```python
from build123d import *

# Parameters (mm, degrees)
SKETCH1_W           = 50.8
SKETCH1_H           = 25.4
BOSS_EXTRUDE1_DEPTH = 2.38125
CUT_EXTRUDE1_REACH  = 6.763
SKETCH2_R           = 3.175


with BuildPart() as part:
    # Sketch1 → Boss-Extrude1 (new body, symmetric)
    with BuildSketch(Plane(origin=(0, 0, 0), x_dir=(1, 0, 0), z_dir=(0, 1, 0))):
        Rectangle(SKETCH1_W, SKETCH1_H)
    extrude(amount=BOSS_EXTRUDE1_DEPTH, both=True)

    # Sketch2 → Cut-Extrude1 (cut, up to next)
    with BuildSketch(Plane(origin=(0, 2.38125, 0), x_dir=(1, 0, 0), z_dir=(0, 1, 0)), mode=Mode.PRIVATE) as cut_extrude1_sk1:
        with Locations((-12.7, 0)):
            Circle(SKETCH2_R)
    cut_extrude1_tool1 = extrude(cut_extrude1_sk1.sketch, amount=-CUT_EXTRUDE1_REACH, mode=Mode.PRIVATE) & part.part
    add(cut_extrude1_tool1.solids().sort_by_distance((-12.7, 2.38125, 0))[0], mode=Mode.SUBTRACT)
    # Sketch2 → Cut-Extrude1 (cut, up to next)
    with BuildSketch(Plane(origin=(0, 2.38125, 0), x_dir=(1, 0, 0), z_dir=(0, 1, 0)), mode=Mode.PRIVATE) as cut_extrude1_sk2:
        with Locations((12.7, 0)):
            Circle(SKETCH2_R)
    cut_extrude1_tool2 = extrude(cut_extrude1_sk2.sketch, amount=-CUT_EXTRUDE1_REACH, mode=Mode.PRIVATE) & part.part
    add(cut_extrude1_tool2.solids().sort_by_distance((12.7, 2.38125, 0))[0], mode=Mode.SUBTRACT)


solid = part.part
```
CAD build for the part. Positions are in the model's coordinates, mm. Coordinates: 2 decimals unless noted, no trailing zeros. Loops run counter-clockwise (first coordinate to the right, second up) from the corner with the lowest first, then second, coordinate; pieces in that order, holes last. Notation, with made-up numbers: (51.5, 50.5) - (95.5, 50.5) arc R24 cw to (95.5, 70.5) - close; hole circle Ø5 at (41.5, 64). An arc over 180 degrees is marked (long way). Return JSON: item names as keys, results as strings.
1. Mould opens along Z. For faces 1 (the flat face through (0, 0, -12.7)), 2 (the cylindrical face through (-9.67, 0.03, -0.95)), 3 (the flat face through (-25.4, 0, 0)), 4 (the cylindrical face through (9.53, 0.03, -0.14)) say: released by +Z, released by -Z, zero draft, split by the parting line, or undercut.
Result:
{"face 1": "released by -Z", "face 2": "undercut", "face 3": "zero draft", "face 4": "undercut"}
2. Band-saw the part on C-C (y = -0.05). Give the cut face in (x, z) (3 decimals), and give its area (3 significant figures).
Result:
{"outline": "(-25.4, -12.7) - (25.4, -12.7) - (25.4, 12.7) - (-25.4, 12.7) - close; hole circle Ø6.35 at (-12.7, 0); hole circle Ø6.35 at (12.7, 0)", "area": "1,230 mm2"}
3. Band-saw the part on A-A (x = -12.7). Give the cut face in (y, z) (3 decimals), and give its area (3 significant figures).
Result:
{"outline": "(-2.381, -12.7) - (2.381, -12.7) - (2.381, -3.175) - (-2.381, -3.175) - close; (-2.381, 3.175) - (2.381, 3.175) - (2.381, 12.7) - (-2.381, 12.7) - close", "area": "90.7 mm2"}
4. Probe L1, parallel to X at y = -0.2, z = 0 (3 decimals); L2, parallel to Z at x = 12.7, y = 1 (3 decimals); L3, parallel to X at y = 1.25, z = 2.25. List the from-to ranges inside material, lowest first. Write a range as from..to.
Result:
{"L1": "x = -25.4..-15.875, -9.525..9.525, 15.875..25.4", "L2": "z = -12.7..-3.175, 3.175..12.7", "L3": "x = -25.4..-14.94, -10.46..10.46, 14.94..25.4"}
5. Band-saw the part on D-D (x = 13). Give the cut face in (y, z).
Result:
{"outline": "(-2.38, -12.7) - (2.38, -12.7) - (2.38, -3.16) - (-2.38, -3.16) - close; (-2.38, 3.16) - (2.38, 3.16) - (2.38, 12.7) - (-2.38, 12.7) - close"}
6. Drop a flat-ended pin along its axis: pin 1 (4 mm diameter, centred on x = -12.7, z = 0, fed in from -Y). Give the stop position or say it passes through.
Result:
{"pin 1": "passes through"}
7. Band-saw the part on B-B (z = 0). Give the cut face in (x, y) (3 decimals).
Result:
{"outline": "(-25.4, -2.381) - (-15.875, -2.381) - (-15.875, 2.381) - (-25.4, 2.381) - close; (-9.525, -2.381) - (9.525, -2.381) - (9.525, 2.381) - (-9.525, 2.381) - close; (15.875, -2.381) - (25.4, -2.381) - (25.4, 2.381) - (15.875, 2.381) - close"}
